Autodesk Fusion 360 part; units mm, degrees
sketch "Sketch1" plane through (0, 0, 0) normal (0, 1, 0) x (1, 0, 0)
  line L0 (0, 0) -> (61, 0)
  line L1 (61, 0) -> (61, -47)
  line L2 (61, -47) -> (0, -47)
  line L3 (0, -47) -> (0, 0)
  circle A0 centre (12, -35) radius 5
  line L4 (0, -16) -> (2.75, -16)
  line L5 (2.75, -16) -> (2.75, -10.55)
  line L6 (2.75, -10.55) -> (0, -10.55)
  line L7 (11.46, 0) -> (11.46, -4.85)
  line L8 (11.46, -4.85) -> (13.91, -4.85)
  line L9 (13.91, -1.85) -> (13.91, -4.85)
  line L10 (18.06, 0) -> (18.06, 4.925)
  line L11 (18.06, 4.925) -> (42.21, 4.925) construction
  line L12 (42.21, 4.925) -> (42.21, 0)
  arc A1 (42.21, 4.925) -> (18.06, 4.925) centre (30.135, 4.925) ccw
  line L13 (45.16, -1.75) -> (45.16, -4.75)
  line L14 (45.16, -4.75) -> (47.61, -4.75)
  line L15 (47.61, -4.75) -> (47.61, 0)
  line L16 (61, -6.3) -> (59.3, -6.3)
  line L17 (59.3, -6.3) -> (59.3, -11.6)
  line L18 (59.3, -11.6) -> (61, -11.6)
  line L19 (61, -25.25) -> (59.3, -25.25)
  line L20 (59.3, -25.25) -> (59.3, -30.55)
  line L21 (59.3, -30.55) -> (61, -30.55)
  line L22 (16, -18.5) -> (38, -18.5)
  line L23 (38, -18.5) -> (38, -4.65)
  line L24 (38, -4.65) -> (16, -4.65)
  line L25 (16, -4.65) -> (16, -18.5)
  circle A2 centre (19.025, -22.5) radius 2.075
  circle A3 centre (33.025, -22.5) radius 2.075
  circle A4 centre (42.7, -20.7) radius 1.5
  circle A5 centre (42.7, -7.4843) radius 1.5
  circle A6 centre (35.8, -43) radius 1.7
  line L26 (13.91, -1.85) -> (18.06, -1.85)
  line L27 (18.06, -1.85) -> (18.06, 0)
  line L28 (30.135, 17) -> (48.0908, 17) construction
  line L29 (42.21, 0) -> (42.21, -1.75)
  line L30 (45.16, -1.75) -> (42.21, -1.75)
  circle A7 centre (49, -35) radius 5
  line L31 (12, -35) -> (49, -35) construction
  line L32 (42.7, -20.7) -> (42.7, -7.4843) construction
  line L33 (9, -45.2) -> (11.2, -45.2)
  line L34 (11.2, -45.2) -> (11.2, -41.9)
  line L35 (11.2, -41.9) -> (9, -41.9)
  line L36 (9, -41.9) -> (9, -45.2)
  line L37 (19.025, -22.5) -> (33.025, -22.5) construction
  circle A8 centre (6, -27) radius 1.5
  circle A9 centre (6, -20) radius 1.5
  line L38 (45.16, 0) -> (45.16, -1.75) construction
  line L39 (13.91, 0) -> (13.91, -1.85) construction
  circle A10 centre (30.135, 4.925) radius 5
  point P0 (6, -27)
  point P1 (6, -20)
  point P2 (12, -35)
  dimension "d1" = 61
  dimension "d2" = 47
  dimension "d3" = 7
  dimension "d4" = 6
  dimension "d5" = 20
  dimension "d20" = 12
  dimension "d21" = 12
  dimension "d22" = 10
  dimension "d25" = 31
  dimension "d26" = 5.45
  dimension "d28" = 2.45
  dimension "d29" = 4.85
  dimension "d30" = 3
  dimension "d32" = 24.15
  dimension "d35" = 11.46
  dimension "d37" = 4.75
  dimension "d38" = 2.45
  dimension "d39" = 13.39
  dimension "d40" = 6.3
  dimension "d41" = 5.3
  dimension "d42" = 1.7
  dimension "d43" = 1.7
  dimension "d44" = 13.65
  dimension "d47" = 5.3
  dimension "d48" = 16.45
  dimension "d49" = 3
  dimension "d50" = 14
  dimension "d51" = 22
  dimension "d52" = 13.85
  dimension "d53" = 16
  dimension "d54" = 4
  dimension "d55" = 10
  dimension "d56" = 12
  dimension "d57" = 25.2
  dimension "d58" = 4
  dimension "d59" = 13.2157
  dimension "d60" = 9
  dimension "d61" = 4.15
  dimension "d62" = 3.4
  dimension "d63" = 3
  dimension "d64" = 3
  dimension "d65" = 6
  dimension "d66" = 20
  dimension "d67" = 3
  dimension "d68" = 18.3
  dimension "d69" = 5.4
  dimension "d70" = 6.6
  dimension "d71" = 26.3
  dimension "d72" = 28.5
  dimension "d73" = 19.025
  dimension "d74" = 10
  dimension "d75" = 3.3
  dimension "d76" = 2.2
  dimension "d77" = 1.8
  dimension "d86" = 2.75
  dimension "d87" = 64
extrude "Extrude1" add sketch "Sketch1" along normal blind 2.75 contours L0 L1 L2 L3 L4 L5 L6 L7 L8 L9 L13 L14 L15 L16 L17 L18 L19 L20 L21 L26 L27 L29 L30 A10 | L0 L10 L12 A1 A10 | L0 A10 | A2 | A3 picked at (30.0387, -0.0222)
extrude "Extrude3" add sketch "Sketch1" against normal blind 5.42 contours A2 | A3
fillet "Fillet1" radius 10 2 edges at (0, 1.375, 47) (61, 1.375, 47)
hole "Hole3" at (19.025, -5.42, 22.5) direction (0, 1, 0) diameter 3 end through all
hole "Hole4" at (33.025, -5.42, 22.5) direction (0, 1, 0) diameter 3 depth 8.17 tip angle 118
thread "Thread1"
thread "Thread2"
thread "Thread3"
thread "Thread4"
thread "Thread5"
thread "Thread6"
extrude "Extrude2" [suppressed]
equation "d71 = 24.8 mm + ( d63 / 2 )"
equation "d73 = 21.1 mm - d61 / 2"
CAD build for the part. Positions are in the model's coordinates, mm. A direction names the side the tool comes from. Give positions to 0.01 mm unless a question says otherwise; leave off trailing zeros. Loops run counter-clockwise (first coordinate to the right, second up) from the corner with the lowest first, then second, coordinate; pieces in that order, holes last. Notation, with made-up numbers: (58.5, -8) -> (86.5, -8) arc R31 cw to (86.5, 31) -> close; hole circle Ø3 at (68.25, 76). An arc over 180 degrees is marked (long way). Use a Markdown table: item, result.
1. Slice it at D-D (y = -1.5). List the corners of the cut face in (x, z) (3 decimals).
Check result:
| item | result |
|---|---|
| outline | circle Ø4.15 at (19.025, 22.5); circle Ø4.15 at (33.025, 22.5); hole circle Ø3 at (19.025, 22.5); hole circle Ø3 at (33.025, 22.5) |
2. Slice it at A-A (z = 13). List the corners of the cut face in (x, y), plus the area to 3 significant figures.
Check result:
| item | result |
|---|---|
| outline | (2.75, 0) -> (16, 0) -> (16, 2.75) -> (2.75, 2.75) -> close; (38, 0) -> (61, 0) -> (61, 2.75) -> (38, 2.75) -> close |
| area | 99.7 mm^2 |
3. Slice it at B-B (z = 35). List the corners of the cut face in (x, y), plus the area to 3 significant figures.
Check result:
| item | result |
|---|---|
| outline | (0, 0) -> (7, 0) -> (7, 2.75) -> (0, 2.75) -> close; (17, 0) -> (44, 0) -> (44, 2.75) -> (17, 2.75) -> close; (54, 0) -> (61, 0) -> (61, 2.75) -> (54, 2.75) -> close |
| area | 113 mm^2 |
4. Mould opens along X. For faces 1 (the cylindrical face through (20.14, -2.67, 20.75)), 2 (the flat face through (30, 1, 0)), 3 (the flat face through (0, 1, 5)), 4 (the flat face through (6, 1, 0)) say: pulls with the +X half, pulls with the -X half, needs draft (parallel to the pull), parting line crosses it, or undercut.
Check result:
| item | result |
|---|---|
| face 1 | undercut |
| face 2 | undercut |
| face 3 | pulls with the -X half |
| face 4 | needs draft |
5. Slice it at C-C (x = 12.5). List the corners of the cut face in (y, z), plus the area to 3 significant figures.
Check result:
| item | result |
|---|---|
| outline | (0, 4.85) -> (2.75, 4.85) -> (2.75, 30.03) -> (0, 30.03) -> close; (0, 39.97) -> (2.75, 39.97) -> (2.75, 47) -> (0, 47) -> close |
| area | 88.6 mm^2 |
6. Which spindle directions (+Z, -Z, +X, -X, +Y, -Y) get a long thin tool onto all of the face, cutting with end or side? Do faces 5 (the flat face through (59.3, 1, 9)), 6 (the flat face through (45.16, 1, 3)), 7 (the flat face through (61, 1, 3)), 8 (the flat face through (2.75, 1, 13)), 9 (the flat face through (10, 1, 41.9)). Say none if no direction does.
Check result:
| item | result |
|---|---|
| face 5 | +X, +Y, -Y |
| face 6 | -Z, +Y, -Y |
| face 7 | +Z, -Z, +X, +Y, -Y |
| face 8 | -X, +Y, -Y |
| face 9 | +Y, -Y |
7. Wall check: L1, parallel to X at y = -2, z = 22.5 (3 decimals); L2, parallel to Z at x = 42.7, y = 0.95; L3, parallel to X at y = -1.5, z = 23. Give the ranges that are in metal, low to high. Write a range as [from, to].
Check result:
| item | result |
|---|---|
| L1 | x = [16.95, 17.525], [20.525, 21.1], [30.95, 31.525], [34.525, 35.1] |
| L2 | z = [1.75, 5.98], [8.98, 19.2], [22.2, 47] |
| L3 | x = [17.01, 17.61], [20.44, 21.04], [31.01, 31.61], [34.44, 35.04] |
8. Flat gauge pins, fed straight in: pin 1 (1.4 mm diameter, centred on y = 2, z = 27, fed in from +X); pin 2 (0.8 mm diameter, centred on x = 15, y = 1.5, fed in from -Z); pin 3 (0.8 mm diameter, centred on x = 2, y = 1.5, fed in from +Z). Where does each tip first touch, or does it go through?
Check result:
| item | result |
|---|---|
| pin 1 | stops at x = 59.3 |
| pin 2 | stops at z = 1.85 |
| pin 3 | stops at z = 43.5 |
